Can you work these out from the model? Positions are in its coordinate system, mm. Face numbers are marked on the shaded views. A direction names the side the tool comes from. Round coordinates to 2 decimals unless told otherwise and drop trailing zeros. Write each loop counter-clockwise with the first axis right and the second up, starting at its lowest first coordinate (ties: lowest second). Pieces come first, ordered by that corner, then holes. Notation, with made-up numbers: (3.5, 11.5) -> (48.5, 11.5) arc R5 ccw to (48.5, 16.5) -> close; hole circle Ø4 at (32, 6). An arc over 180 degrees is marked (long way). Write item = value, one per line. Start each with the question number.
1) Thinking about a two-plate mould opening in X: for the marked faces 1, 2, 3 and 4, which applies, +X half, -X half, draft (parallel to the pull), parting line (faces both ways), or undercut?
2) For the marked faces 5, 6, 7 and 8, which set-ups out of +Z, -Z, +X, -X, +Y, -Y let a thin tool reach every point of the face, with its end or its side?
3) Imagine slicing it at A-A, the plane y = 8.5. Please give me the cut outline in (x, z).
4) Imagine slicing it at B-B, the plane x = 10.5. Please give me the cut outline in (y, z).
5) If I drill on line 1 (X direction, y = 3.75, z = 6); line 2 (X direction, y = 7, z = 3.5); line 3 (Y direction, x = 5.25, z = 9), over which ranges is the centre line in solid material (lowest first)?
6) Imagine slicing it at D-D, the plane y = 1.25. Please give me the cut outline in (x, z), then the cut area to 3 significant figures.
7) Imagine slicing it at C-C, the plane z = 7.5. Please give me the cut outline in (x, y), then the cut area to 3 significant figures.
8) I'm going to push flat-ended pins straight in: pin 1 (2 mm diameter, centred on x = 11, z = 6, fed in from +Y); pin 2 (1 mm diameter, centred on y = 12.5, z = 6, fed in from +X); pin 3 (5 mm diameter, centred on x = -4.5, y = 1.5, fed in from -Z); pin 4 (3.5 mm diameter, centred on x = -2, z = 5, fed in from +Y). Where does each tip first touch, or does it pass through?
from build123d import *

# Parameters (mm, degrees)
F0_W        = 6
F0_H        = 0.95
F1_DEPTH    = 11
F2_C1_SIZE  = 1
F2_C2_SIZE  = 1
F2_C3_SIZE  = 1
F2_C4_SIZE  = 1
F2_C5_SIZE  = 1
F2_C6_SIZE  = 1
F2_C7_SIZE  = 1
F2_C8_SIZE  = 1
F2_C9_SIZE  = 1
F2_C10_SIZE = 1
F2_C11_SIZE = 1
F2_C12_SIZE = 0.9999
F2_C13_SIZE = 1
F2_C14_SIZE = 1
F3_C1_SIZE  = 1
F3_C2_SIZE  = 1
F3_C3_SIZE  = 1
F3_C4_SIZE  = 1
F3_C5_SIZE  = 1
F3_C6_SIZE  = 0.9999
F3_C7_SIZE  = 1
F3_C8_SIZE  = 1
F3_C9_SIZE  = 1
F3_C10_SIZE = 1
F3_C11_SIZE = 1
F3_C12_SIZE = 1
F3_C13_SIZE = 1
F3_C14_SIZE = 1


# Not quite as in the source:
# - a fillet or chamfer is up to 0.001 mm smaller than in the source, because OpenCascade refuses the exact size


with BuildPart() as f1:
    # F0 (on Top) → F1 (new body)
    with BuildSketch(Plane.XY):
        Polygon((0.25, 10.5), (0, 0), (-4.546, 0), (-8.77, 0), (-7.546, 5.4), (-6.05, 12), (-12.05, 12), (-12.05, -4), (15.95, -4), (15.95, 10.5), (8.65, 10.5), (8.65, 0), (5.75, 0), (5.75, 10.5), align=None)
        Polygon((-8.77, 0), (-4.546, 0), (-4.546, 5.4), (-7.546, 5.4), align=None)
        with Locations((-9.05, 12.475)):
            Rectangle(F0_W, F0_H)
    extrude(amount=F1_DEPTH)

    # F2: chamfer of 1 on 14 edges, made by hand

    # F2_c1
    f2_c1_edges = [f1.edges().sort_by_distance(p)[0] for p in [
        (0.125, 5.25, 11),
    ]]
    chamfer(f2_c1_edges, length=F2_C1_SIZE)

    # F2_c2
    f2_c2_edges = [f1.edges().sort_by_distance(p)[0] for p in [
        (-2.273, 0, 11),
    ]]
    chamfer(f2_c2_edges, length=F2_C2_SIZE)

    # F2_c3
    f2_c3_edges = [f1.edges().sort_by_distance(p)[0] for p in [
        (-4.546, 2.7, 11),
    ]]
    chamfer(f2_c3_edges, length=F2_C3_SIZE)

    # F2_c4
    f2_c4_edges = [f1.edges().sort_by_distance(p)[0] for p in [
        (-6.546, 5.4, 11),
    ]]
    chamfer(f2_c4_edges, length=F2_C4_SIZE)

    # F2_c5
    f2_c5_edges = [f1.edges().sort_by_distance(p)[0] for p in [
        (-6.798, 8.7, 11),
    ]]
    chamfer(f2_c5_edges, length=F2_C5_SIZE)

    # F2_c6
    f2_c6_edges = [f1.edges().sort_by_distance(p)[0] for p in [
        (-9.4550169048, 12.95, 11),
    ]]
    chamfer(f2_c6_edges, length=F2_C6_SIZE)

    # F2_c7
    f2_c7_edges = [f1.edges().sort_by_distance(p)[0] for p in [
        (-12.05, 3.975, 11),
    ]]
    chamfer(f2_c7_edges, length=F2_C7_SIZE)

    # F2_c8
    f2_c8_edges = [f1.edges().sort_by_distance(p)[0] for p in [
        (2.45, -4, 11),
    ]]
    chamfer(f2_c8_edges, length=F2_C8_SIZE)

    # F2_c9
    f2_c9_edges = [f1.edges().sort_by_distance(p)[0] for p in [
        (15.95, 3.75, 11),
    ]]
    chamfer(f2_c9_edges, length=F2_C9_SIZE)

    # F2_c10
    f2_c10_edges = [f1.edges().sort_by_distance(p)[0] for p in [
        (11.8, 10.5, 11),
    ]]
    chamfer(f2_c10_edges, length=F2_C10_SIZE)

    # F2_c11
    f2_c11_edges = [f1.edges().sort_by_distance(p)[0] for p in [
        (8.65, 4.75, 11),
    ]]
    chamfer(f2_c11_edges, length=F2_C11_SIZE)

    # F2_c12 (size 1 in the source; OpenCascade refuses exactly that, so slightly less here)
    f2_c12_edges = [f1.edges().sort_by_distance(p)[0] for p in [
        (7.2, 0, 11),
    ]]
    chamfer(f2_c12_edges, length=F2_C12_SIZE)

    # F2_c13
    f2_c13_edges = [f1.edges().sort_by_distance(p)[0] for p in [
        (5.75, 5.25, 11),
    ]]
    chamfer(f2_c13_edges, length=F2_C13_SIZE)

    # F2_c14
    f2_c14_edges = [f1.edges().sort_by_distance(p)[0] for p in [
        (3.0001417033, 10.5, 11),
    ]]
    chamfer(f2_c14_edges, length=F2_C14_SIZE)

    # F3: chamfer of 1 on 14 edges, made by hand

    # F3_c1
    f3_c1_edges = [f1.edges().sort_by_distance(p)[0] for p in [
        (5.75, 5.25, 0),
    ]]
    chamfer(f3_c1_edges, length=F3_C1_SIZE)

    # F3_c2
    f3_c2_edges = [f1.edges().sort_by_distance(p)[0] for p in [
        (7.2, 0, 0),
    ]]
    chamfer(f3_c2_edges, length=F3_C2_SIZE)

    # F3_c3
    f3_c3_edges = [f1.edges().sort_by_distance(p)[0] for p in [
        (2.5, 10.5, 0),
    ]]
    chamfer(f3_c3_edges, length=F3_C3_SIZE)

    # F3_c4
    f3_c4_edges = [f1.edges().sort_by_distance(p)[0] for p in [
        (0.1130952381, 4.75, 0),
    ]]
    chamfer(f3_c4_edges, length=F3_C4_SIZE)

    # F3_c5
    f3_c5_edges = [f1.edges().sort_by_distance(p)[0] for p in [
        (8.65, 5.25, 0),
    ]]
    chamfer(f3_c5_edges, length=F3_C5_SIZE)

    # F3_c6 (size 1 in the source; OpenCascade refuses exactly that, so slightly less here)
    f3_c6_edges = [f1.edges().sort_by_distance(p)[0] for p in [
        (-2.273, 0, 0),
    ]]
    chamfer(f3_c6_edges, length=F3_C6_SIZE)

    # F3_c7
    f3_c7_edges = [f1.edges().sort_by_distance(p)[0] for p in [
        (12.8, 10.5, 0),
    ]]
    chamfer(f3_c7_edges, length=F3_C7_SIZE)

    # F3_c8
    f3_c8_edges = [f1.edges().sort_by_distance(p)[0] for p in [
        (15.95, 2.75, 0),
    ]]
    chamfer(f3_c8_edges, length=F3_C8_SIZE)

    # F3_c9
    f3_c9_edges = [f1.edges().sort_by_distance(p)[0] for p in [
        (-4.546, 2.7, 0),
    ]]
    chamfer(f3_c9_edges, length=F3_C9_SIZE)

    # F3_c10
    f3_c10_edges = [f1.edges().sort_by_distance(p)[0] for p in [
        (1.45, -4, 0),
    ]]
    chamfer(f3_c10_edges, length=F3_C10_SIZE)

    # F3_c11
    f3_c11_edges = [f1.edges().sort_by_distance(p)[0] for p in [
        (-6.546, 5.4, 0),
    ]]
    chamfer(f3_c11_edges, length=F3_C11_SIZE)

    # F3_c12
    f3_c12_edges = [f1.edges().sort_by_distance(p)[0] for p in [
        (-12.05, 4.975, 0),
    ]]
    chamfer(f3_c12_edges, length=F3_C12_SIZE)

    # F3_c13
    f3_c13_edges = [f1.edges().sort_by_distance(p)[0] for p in [
        (-8.55, 12.95, 0),
    ]]
    chamfer(f3_c13_edges, length=F3_C13_SIZE)

    # F3_c14
    f3_c14_edges = [f1.edges().sort_by_distance(p)[0] for p in [
        (-6.8036666667, 8.675, 0),
    ]]
    chamfer(f3_c14_edges, length=F3_C14_SIZE)


solid = f1.part
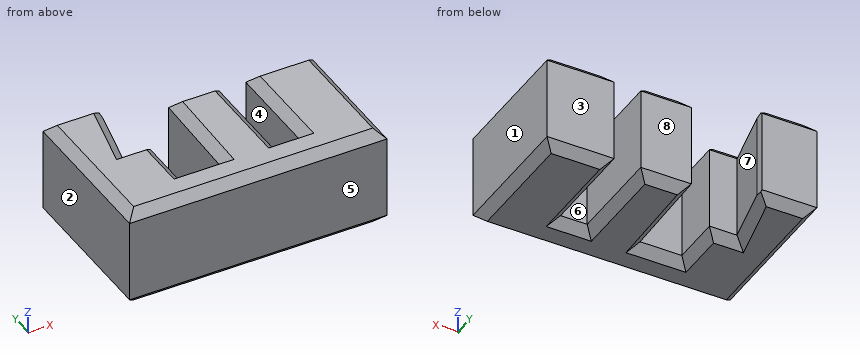
Reported:
q1.face_1 = +X half
q1.face_2 = -X half
q1.face_3 = draft
q1.face_4 = undercut
q2.face_5 = +Z, -Z, +X, -X, -Y
q2.face_6 = +Z, -Z, +Y
q2.face_7 = +Z, -Z
q2.face_8 = +Z, -Z, +X, +Y
q3.outline = (-12.05, 1) -> (-11.05, 0) -> (-7.87, 0) -> (-6.84, 1) -> (-6.84, 10) -> (-7.87, 11) -> (-11.05, 11) -> (-12.05, 10) -> close; (0.2, 1) -> (1.2, 0) -> (4.75, 0) -> (5.75, 1) -> (5.75, 10) -> (4.75, 11) -> (1.2, 11) -> (0.2, 10) -> close; (8.65, 1) -> (9.65, 0) -> (14.95, 0) -> (15.95, 1) -> (15.95, 10) -> (14.95, 11) -> (9.65, 11) -> (8.65, 10) -> close
q4.outline = (-4, 1) -> (-3, 0) -> (9.5, 0) -> (10.5, 1) -> (10.5, 10) -> (9.5, 11) -> (-3, 11) -> (-4, 10) -> close
q5.line_1 = -12.05 to -4.55, 0.09 to 5.75, 8.65 to 15.95
q5.line_2 = -12.05 to -7.18, 0.17 to 5.75, 8.65 to 15.95
q5.line_3 = -4 to 10.5
q6.outline = (-12.05, 1) -> (-11.05, 0) -> (-5.55, 0) -> (-4.55, 1) -> (-4.55, 10) -> (-5.55, 11) -> (-11.05, 11) -> (-12.05, 10) -> close; (0.03, 1) -> (1.03, 0) -> (4.75, 0) -> (5.75, 1) -> (5.75, 10) -> (4.75, 11) -> (1.03, 11) -> (0.03, 10) -> close; (8.65, 1) -> (9.65, 0) -> (14.95, 0) -> (15.95, 1) -> (15.95, 10) -> (14.95, 11) -> (9.65, 11) -> (8.65, 10) -> close
q6.area = 220 mm²
q7.outline = (-12.05, -4) -> (15.95, -4) -> (15.95, 10.5) -> (8.65, 10.5) -> (8.65, 0) -> (5.75, 0) -> (5.75, 10.5) -> (0.25, 10.5) -> (0, 0) -> (-4.55, 0) -> (-4.55, 5.4) -> (-7.55, 5.4) -> (-6.05, 12) -> (-6.05, 12.95) -> (-12.05, 12.95) -> close
q7.area = 329 mm²
q8.pin_1 = 10.5
q8.pin_2 = -6.05
q8.pin_3 = 0
q8.pin_4 = 0
